Read the model definition and answer for the solid it produces. Units are mm, in the model's axes. A direction names the side the tool comes from. Give positions to 0.01 mm unless a question says otherwise; leave off trailing zeros. Loops run counter-clockwise (first coordinate to the right, second up) from the corner with the lowest first, then second, coordinate; pieces in that order, holes last. Notation, with made-up numbers: (20, 15.5) - (29, 15.5) arc R16 ccw to (29, 32.5) - close; hole circle Ø5 at (-37.5, -14.75). An arc over 180 degrees is marked (long way). Write item = value, one per line.
```python
from build123d import *

# Parameters (mm, degrees)
F7_W      = 2.55
F7_H      = 4.1
F7_W_2    = 1.55
F7_H_2    = 3.1
F6_R      = 9.525
F6_W      = 4.1
F6_H      = 2.55
F9_DEPTH  = 6.35
F7_R      = 9.525
F10_DEPTH = 6.35


with BuildPart() as f8:
    # F8: sweep along a path in F4, F2, F0
    with BuildLine(Plane.YZ.offset(-82)) as f8_path:
        Line((0, -92), (-10, -92))
        ThreePointArc((-10, -92), (-20.8894444303, -87.4894444303), (-25.4, -76.6))
        Line((-25.4, -76.6), (-25.4, -66.6))
    with BuildLine(Plane.XZ.offset(25.4)) as f8_path_2:
        Line((-82, -66.6), (-82, -25.4))
        Line((-82, -25.4), (-82, -15.4))
        ThreePointArc((-82, -15.4), (-77.4894444303, -4.5105555697), (-66.6, 0))
        Line((-66.6, 0), (-56.6, 0))
    with BuildLine(Plane.XY) as f8_path_3:
        Line((-56.6, -25.4), (-25.4, -25.4))
        Line((-25.4, -25.4), (-15.4, -25.4))
        ThreePointArc((-15.4, -25.4), (-4.5105555697, -20.8894444303), (0, -10))
        Line((0, -10), (0, 0))
        Line((0, 0), (0, 33))
    # F7 (on Front) → F8 (sweep)
    with BuildSketch(Plane.XZ):
        with Locations((-82, -92)):
            Rectangle(F7_W, F7_H)
        with Locations((-82, -92)):
            Rectangle(F7_W_2, F7_H_2, mode=Mode.SUBTRACT)
    sweep(path=f8_path.line + f8_path_2.line + f8_path_3.line)

    # F6 (on offset) → F9 (join)
    with BuildSketch(Plane.XZ.offset(-33)):
        Circle(F6_R)
        Rectangle(F6_W, F6_H, mode=Mode.SUBTRACT)
    extrude(amount=F9_DEPTH)

    # F7 (on Front) → F10 (join)
    with BuildSketch(Plane.XZ):
        with Locations((-82, -92)):
            Circle(F7_R)
        with Locations((-82, -92)):
            Rectangle(F7_W, F7_H, mode=Mode.SUBTRACT)
    extrude(amount=F10_DEPTH)


solid = f8.part
```
1) Find the intervals of material crossed by probe 1 along Y at (x, z) = (-60, -0.5); probe 2 along Y at (x, z) = (-73.5, -90); probe 3 along X at (y, z) = (29.5, -5.5), in increasing order.
Output:
probe_1 = -27.45 to -26.95, -23.85 to -23.35
probe_2 = -6.35 to 0
probe_3 = -7.78 to 7.78
2) The mould has two halves that part along X. Classify faces 1 (the face through (2.05, 9, 0)), 2 (the face through (-12, -24, 0.775)), 3 (the face through (-82, -27.45, -20)): pulls with the +X half, pulls with the -X half, needs draft (parallel to the pull), parting line crosses it, or undercut.
Output:
face_1 = pulls with the +X half
face_2 = undercut
face_3 = needs draft
3) A tool of negligible diameter and unlimited length cuts with its end or side. For faces 4 (the face through (-5.715, -19.901, -0.011)), 5 (the face through (-82.02, -19.34, -86.14)), 6 (the face through (-82, -23.35, -20)), 7 (the face through (-19, -24, 1.275)), from which of +Z, -Z, +X, -X, +Y, -Y can it reach the whole face along a straight path? Write none if from no direction.
Output:
face_4 = none
face_5 = +Z, +X, -X
face_6 = +Z, -X, +Y
face_7 = +Z, +X, -X, -Y
4) Each of these flat-tipped pins is pushed along its axis until it touches: P1, Ø12, axis at y = 22, z = -11, coming from the +X side; P2, Ø12, axis at y = -14.5, z = -6.5, coming from the +X side; P3, Ø1.3, axis at x = -82, y = -8, coming from the -Z side. Where does it stop, or does it pass through?
Output:
P1 = 6.23
P2 = 1.98
P3 = -94.05
5) A cutting plane is placed at A-A on y = -2.5. Determine the outline of the cut face in (x, z) (3 decimals), then the cut area to 3 significant figures.
Output:
outline = circle Ø19.05 at (-82, -92); (-2.05, -1.275) - (2.05, -1.275) - (2.05, 1.275) - (-2.05, 1.275) - close; hole (-82.775, -93.55) - (-81.225, -93.55) - (-81.225, -90.45) - (-82.775, -90.45) - close; hole (-1.55, -0.775) - (1.55, -0.775) - (1.55, 0.775) - (-1.55, 0.775) - close
area = 286 mm²
6) A cutting plane is placed at B-B on x = -44. Determine the outline of the cut face in (y, z) (3 decimals), then the cut area to 3 significant figures.
Output:
outline = (-27.45, -1.275) - (-23.35, -1.275) - (-23.35, 1.275) - (-27.45, 1.275) - close; hole (-26.95, -0.775) - (-23.85, -0.775) - (-23.85, 0.775) - (-26.95, 0.775) - close
area = 5.65 mm²
7) A cutting plane is placed at C-C on z = -3.5. Determine the outline of the cut face in (x, y), then the cut area to 3 significant figures.
Output:
outline = (-78.28, -27.45) - (-74.21, -27.45) - (-74.21, -23.35) - (-78.28, -23.35) - close; (-8.86, 26.65) - (8.86, 26.65) - (8.86, 33) - (-8.86, 33) - close; hole (-77.56, -26.95) - (-75.1, -26.95) - (-75.1, -23.85) - (-77.56, -23.85) - close
area = 122 mm²
8) A cutting plane is placed at D-D on x = -75.5. Determine the outline of the cut face in (y, z), then the cut area to 3 significant figures.
Output:
outline = (-27.45, -4.43) - (-23.35, -4.43) - (-23.35, -1.3) - (-27.45, -1.3) - close; (-6.35, -98.96) - (0, -98.96) - (0, -85.04) - (-6.35, -85.04) - close; hole (-26.95, -3.79) - (-23.85, -3.79) - (-23.85, -1.89) - (-26.95, -1.89) - close
area = 95.4 mm²
